from build123d import *

# Parameters (mm, degrees)
F0_W     = 22.479
F0_H     = 13.97
F1_DEPTH = 10.033
F2_W     = 5.1435
F2_H     = 5.08
F2_R     = 1.016
F3_DEPTH = 1.1684
F4_W     = 0.82242
F4_H     = 0.767591
F5_DEPTH = 1.27


with BuildPart() as f1:
    # F0 (on Top) → F1 (new body)
    with BuildSketch(Plane.XY):
        with Locations((11.2395, 6.985)):
            Rectangle(F0_W, F0_H)
    extrude(amount=F1_DEPTH)

    # F2 (on face) → F3 (join)
    with BuildSketch(Plane(origin=(0, 0, 0), x_dir=(1, 0, 0), z_dir=(0, 0, -1))):
        with Locations((-2.57175, -6.985)):
            Rectangle(F2_W, F2_H)
        with Locations((-2.57175, -6.985)):
            Circle(F2_R, mode=Mode.SUBTRACT)
        with Locations((25.05075, -6.985)):
            Rectangle(F2_W, F2_H)
        with Locations((25.05075, -6.985)):
            Circle(F2_R, mode=Mode.SUBTRACT)
    extrude(amount=-F3_DEPTH)

    # F4 (on face) → F5 (cut)
    with BuildSketch(Plane.XY.offset(10.033)):
        Polygon((13.786751, 10.79755), (13.786751, 10.982947), (9.691444, 10.982947), (10.554357, 10.241496), (13.258331, 10.241496), align=None)
        Polygon((10.425497, 10.104383), (9.64253, 10.777142), (9.64253, 6.367391), (10.425497, 6.807481), align=None)
        Polygon((9.767849, 6.309171), (10.425497, 6.003647), (12.916651, 6.003647), (13.521753, 6.435402), (12.894051, 6.807481), (10.648357, 6.807481), align=None)
        Polygon((13.786751, 1.735938), (13.786751, 6.003647), (13.786751, 6.405564), (12.916651, 5.813658), (12.916651, 2.628638), align=None)
        Polygon((10.011367, 1.583957), (13.558927, 1.583957), (12.718385, 2.407485), (10.674233, 2.407485), align=None)
        with Locations((15.336972, 1.578371)):
            Rectangle(F4_W, F4_H)
        Polygon((20.461116, 6.582137), (18.215422, 6.582137), (17.587719, 6.210058), (18.192822, 5.778302), (20.683976, 5.778302), (21.341624, 6.083827), align=None)
        Polygon((17.322722, 10.572206), (17.851142, 10.016152), (20.555116, 10.016152), (21.418029, 10.757603), (17.322722, 10.757603), align=None)
        Polygon((20.683976, 9.879039), (20.683976, 6.582137), (21.466942, 6.142047), (21.466942, 10.551798), align=None)
        Polygon((17.322722, 1.510594), (18.192822, 2.403293), (18.192822, 5.588314), (17.322722, 6.18022), align=None)
        Polygon((21.098106, 1.358613), (20.43524, 2.182141), (18.391088, 2.182141), (17.550545, 1.358613), align=None)
    extrude(amount=-F5_DEPTH, mode=Mode.SUBTRACT)


solid = f1.part
Read the model definition and answer for the solid it produces. Units are mm, in the model's axes. A direction names the side the tool comes from. Coordinates: 2 decimals unless noted, no trailing zeros. Loops run counter-clockwise (first coordinate to the right, second up) from the corner with the lowest first, then second, coordinate; pieces in that order, holes last. Notation, with made-up numbers: (-7.75, 78) - (14.25, 78) arc R18 ccw to (14.25, 107) - close; hole circle Ø10 at (79.5, -26.5). An arc over 180 degrees is marked (long way). Answer in a Markdown table with one row per item.
Q1. Find section C-C on z = 9.5. Count the separate pieces of the cut face and the enclosed holes in it, plus the area to 3 significant figures.
Here are the results:
| item | result |
|---|---|
| separate pieces | 1 |
| enclosed holes | 11 |
| area | 286 mm^2 |
Q2. Given P1, Ø3, axis at x = 19, y = 2, coming from the +Z side; P2, Ø0.6, axis at y = 1.5, z = 9.5, coming from the -X side; P3, Ø1.3, axis at x = -2.5, z = 1, coming from the -Y side (3 decimals); P4, Ø5, axis at y = 4, z = 5.5, coming from the +X side, each flat-ended and moving along its own axis, determine where each tip first touches the part or whether it passes through.
Here are the results:
| item | result |
|---|---|
| P1 | stops at z = 10.03 |
| P2 | stops at x = 0 |
| P3 | stops at y = 4.445 |
| P4 | stops at x = 22.48 |
Q3. For faces 4 (the flat face through (19, 10.758, 9)), 5 (the flat face through (-2.6, 5.8, 1.168)), 6 (the flat face through (11, 7, 10.033)), determine the directions among +Z, -Z, +X, -X, +Y, -Y from which every point of the face is accessible in a straight line to the end or side of a thin tool.
Here are the results:
| item | result |
|---|---|
| face 4 | +Z |
| face 5 | +Z, -X, +Y, -Y |
| face 6 | +Z, +X, -X, +Y, -Y |
Q4. Straight lines are drawn through the part: line 1 along X through (y, z) = (11, 1.75); line 2 along Z through (x, y) = (11, 2.25). For each, find the intervals that lie inside material, in ascending order. Write a range as [from, to].
Here are the results:
| item | result |
|---|---|
| line 1 | x = [0, 22.48] |
| line 2 | z = [0, 8.76] |
Q5. Find section B-B on y = 8.75. Write down the section's boundary in (x, z).
Here are the results:
| item | result |
|---|---|
| outline | (-5.14, 0) - (27.62, 0) - (27.62, 1.17) - (22.48, 1.17) - (22.48, 10.03) - (21.47, 10.03) - (21.47, 8.76) - (20.68, 8.76) - (20.68, 10.03) - (10.43, 10.03) - (10.43, 8.76) - (9.64, 8.76) - (9.64, 10.03) - (0, 10.03) - (0, 1.17) - (-5.14, 1.17) - close |
Q6. Find section A-A on x = 19. Write down the section's boundary in (y, z), plus the area to 3 significant figures.
Here are the results:
| item | result |
|---|---|
| outline | (0, 0) - (13.97, 0) - (13.97, 10.03) - (10.76, 10.03) - (10.76, 8.76) - (10.02, 8.76) - (10.02, 10.03) - (6.58, 10.03) - (6.58, 8.76) - (5.78, 8.76) - (5.78, 10.03) - (2.18, 10.03) - (2.18, 8.76) - (1.36, 8.76) - (1.36, 10.03) - (0, 10.03) - close |
| area | 137 mm^2 |
Q7. The mould has two halves that part along X. Classify faces 1 (the flat face through (25, 4.445, 1)), 2 (the flat face through (27.623, 7, 1)), 3 (the flat face through (17.323, 4, 9)): pulls with the +X half, pulls with the -X half, needs draft (parallel to the pull), parting line crosses it, or undercut.
Here are the results:
| item | result |
|---|---|
| face 1 | needs draft |
| face 2 | pulls with the +X half |
| face 3 | undercut |
Q8. Find section D-D on z = 6.25. Write down the section's boundary in (x, y), plus the area to 3 significant figures.
Here are the results:
| item | result |
|---|---|
| outline | (0, 0) - (22.48, 0) - (22.48, 13.97) - (0, 13.97) - close |
| area | 314 mm^2 |
